```python
from build123d import *

# Parameters (mm, degrees)
SKETCH1_R            = 3.75
SKETCH1_R_2          = 2.7
BOSS_EXTRUDE1_DEPTH  = 15
BOSS_EXTRUDE7_START  = -3.75
SKETCH4_R            = 3.75
SKETCH4_R_2          = 2.7
BOSS_EXTRUDE7_DEPTH  = 15
SKETCH5_R            = 2.7
CUT_EXTRUDE1_DEPTH   = 15
SKETCH9_R            = 2.7
BOSS_EXTRUDE11_DEPTH = 1
SKETCH10_R           = 2.7
BOSS_EXTRUDE12_DEPTH = 1
CUT_EXTRUDE10_START  = -12
SKETCH11_R           = 2.7
CUT_EXTRUDE10_DEPTH  = 12
CUT_EXTRUDE11_START  = -12
SKETCH13_R           = 2.7
CUT_EXTRUDE11_DEPTH  = 12
CUT_EXTRUDE2_START   = 3.75
SKETCH6_R            = 2.7
CUT_EXTRUDE2_DEPTH   = 15
SKETCH8_R            = 2.7
BOSS_EXTRUDE9_DEPTH  = 1


with BuildPart() as part:
    # Sketch1 → Boss-Extrude1 (new body)
    with BuildSketch(Plane.XY):
        Circle(SKETCH1_R)
        Circle(SKETCH1_R_2, mode=Mode.SUBTRACT)
    extrude(amount=BOSS_EXTRUDE1_DEPTH)

    # Sketch4 → Boss-Extrude7 (add)
    with BuildSketch(Plane(origin=(0, 0, 0), x_dir=(1, 0, 0), z_dir=(0, 1, 0)).offset(BOSS_EXTRUDE7_START)):
        with Locations(Location((0, -3.75, 0), (0, 0, 90))):
            Circle(SKETCH4_R)
        with Locations(Location((0, -3.75, 0), (0, 0, 90))):
            Circle(SKETCH4_R_2, mode=Mode.SUBTRACT)
    extrude(amount=BOSS_EXTRUDE7_DEPTH)

    # Sketch5 → Cut-Extrude1 (cut)
    with BuildSketch(Plane(origin=(0, 0, 0), x_dir=(1, 0, 0), z_dir=(0, 1, 0))):
        with Locations((0, -3.75)):
            Circle(SKETCH5_R)
    extrude(amount=CUT_EXTRUDE1_DEPTH, mode=Mode.SUBTRACT)

    # Sketch9 → Boss-Extrude11 (add)
    with BuildSketch(Plane.XZ.offset(3.75)):
        with Locations((0, 3.75)):
            Circle(SKETCH9_R)
    extrude(amount=-BOSS_EXTRUDE11_DEPTH)

    # Sketch10 → Boss-Extrude12 (add)
    with BuildSketch(Plane(origin=(0, 0, 0), x_dir=(-1, 0, 0), z_dir=(0, 0, -1))):
        Circle(SKETCH10_R)
    extrude(amount=-BOSS_EXTRUDE12_DEPTH)

    # Sketch11 → Cut-Extrude10 (cut)
    with BuildSketch(Plane(origin=(0, 11.25, 0), x_dir=(1, 0, 0), z_dir=(0, 1, 0)).offset(CUT_EXTRUDE10_START)):
        with Locations(Location((0, -3.75, 0), (0, 0, 163.872379787))):
            Circle(SKETCH11_R)
    extrude(amount=CUT_EXTRUDE10_DEPTH, mode=Mode.SUBTRACT)

    # Sketch13 → Cut-Extrude11 (cut)
    with BuildSketch(Plane.XY.offset(15).offset(CUT_EXTRUDE11_START)):
        Circle(SKETCH13_R)
    extrude(amount=CUT_EXTRUDE11_DEPTH, mode=Mode.SUBTRACT)

    # Sketch6 → Cut-Extrude2 (cut)
    with BuildSketch(Plane.XY.offset(CUT_EXTRUDE2_START)):
        Circle(SKETCH6_R)
    extrude(amount=CUT_EXTRUDE2_DEPTH, mode=Mode.SUBTRACT)

    # Sketch8 → Boss-Extrude9 (add)
    with BuildSketch(Plane(origin=(0, 0, 0), x_dir=(-1, 0, 0), z_dir=(0, 0, -1))):
        with Locations(Location((0, 0, 0), (0, 0, 180))):
            Circle(SKETCH8_R)
    extrude(amount=-BOSS_EXTRUDE9_DEPTH)


solid = part.part
```
Geometry: final body of the model. Coordinates: model frame, mm. A direction names the side the tool comes from. Round coordinates to 2 decimals unless told otherwise and drop trailing zeros. Loops run counter-clockwise (first coordinate to the right, second up) from the corner with the lowest first, then second, coordinate; pieces in that order, holes last. Notation, with made-up numbers: (1, 0.5) -> (18, 0.5) arc R5 ccw to (18, 7.5) -> close; hole circle Ø2 at (-21.5, 12.25). An arc over 180 degrees is marked (long way). Use one line per item in the form item = value.
Item 1: Material intervals for probe 1 along Y at (x, z) = (0, 9.5); probe 2 along Y at (x, z) = (0, 5.25), sorted ascending.
Evaluation:
probe_1 = -3.75 to -2.7, 2.7 to 3.75
probe_2 = -3.75 to -2.7
Item 2: Cut plane B-B on y = 8.75. Output: boundary loops of the cut face in (x, z).
Evaluation:
outline = circle Ø7.5 at (0, 3.75); hole circle Ø5.4 at (0, 3.75)
Item 3: Contact query for flat-ended pins moving along their axis: pin 1 Ø6 at (y, z) = (0.5, 11) entering from -X; pin 2 Ø3 at (x, y) = (0, 0) entering from +Z (3 decimals); pin 3 Ø1 at (y, z) = (9, 9.5) entering from +X; pin 4 Ø2 at (x, y) = (2, 8.5) entering from -Z. Output: stop coordinate, or through.
Evaluation:
pin_1 = -3.75
pin_2 = 1.505
pin_3 = through
pin_4 = 0.14
Item 4: Cut plane C-C on z = 14. Output: boundary loops of the cut face in (x, y), then the cut area to 3 significant figures.
Evaluation:
outline = circle Ø7.5 at (0, 0); hole circle Ø5.4 at (0, 0)
area = 21.3 mm2
Item 5: Cut plane A-A on x = -0.75. Output: boundary loops of the cut face in (y, z), then the cut area to 3 significant figures.
Evaluation:
outline = (-3.75, 0.08) -> (-3.67, 0.08) -> (-3.67, 0) -> (3.67, 0) -> (3.67, 0.08) -> (11.25, 0.08) -> (11.25, 1.16) -> (-2.59, 1.16) -> (-2.59, 15) -> (-3.67, 15) -> (-3.67, 7.42) -> (-3.75, 7.42) -> close; (2.59, 6.34) -> (11.25, 6.34) -> (11.25, 7.42) -> (3.67, 7.42) -> (3.67, 15) -> (2.59, 15) -> close
area = 49.7 mm2
Item 6: Access query for faces 4 (the cylindrical face through (-3.746, 0.165, 10.546)), 5 (the cylindrical face through (-3.75, 0.03, 1.03)), 6 (the cylindrical face through (-0.165, 6.796, 7.496)). Directions: +Z, -Z, +X, -X, +Y, -Y. A direction counts if a zero-diameter tool reaches every point of the face in a straight line with its end or side. Return the directions, or none.
Evaluation:
face_4 = +Z
face_5 = -Z, -X
face_6 = +Y
Item 7: Draft query along Z for faces 1 (the flat face through (0, 0, 0)), 2 (the flat face through (0, -3.75, 4)), 3 (the cylindrical face through (-3.75, -2.72, 3.72)). Return one class per face: released by +Z, released by -Z, zero draft, split by the parting line, or undercut.
Evaluation:
face_1 = released by -Z
face_2 = zero draft
face_3 = split by the parting line
